Autodesk Inventor part; units mm, degrees
ref_plane "YZ Plane" through (0, 0, 0) normal (1, 0, 0) x (0, 1, 0)
ref_plane "XZ Plane" through (0, 0, 0) normal (0, 1, 0) x (-1, 0, 0)
ref_plane "XY Plane" through (0, 0, 0) normal (0, 0, 1) x (1, 0, 0)
sketch "Sketch1" plane through (0, 0, 0) normal (0, 1, 0) x (-1, 0, 0)
  line L0 (59.9595, 0.0507) -> (-0.0405, 0.0507)
  line L1 (-0.0405, 0.0507) -> (-0.0405, -59.9493)
  line L2 (-0.0405, -59.9493) -> (59.9595, -59.9493)
  line L3 (59.9595, -59.9493) -> (59.9595, 0.0507)
  line L4 (54, -52.088) -> (6, -52.088)
  line L5 (6, -52.088) -> (6, -50.088)
  line L6 (6, -50.088) -> (54, -50.088)
  line L7 (54, -50.088) -> (54, -52.088)
  line L8 (54, -46.088) -> (6, -46.088)
  line L9 (6, -46.088) -> (6, -44.088)
  line L10 (6, -44.088) -> (54, -44.088)
  line L11 (54, -44.088) -> (54, -46.088)
  line L12 (54, -40.088) -> (6, -40.088)
  line L13 (6, -40.088) -> (6, -38.088)
  line L14 (6, -38.088) -> (54, -38.088)
  line L15 (54, -38.088) -> (54, -40.088)
  line L16 (54, -34.088) -> (6, -34.088)
  line L17 (6, -34.088) -> (6, -32.088)
  line L18 (6, -32.088) -> (54, -32.088)
  line L19 (54, -32.088) -> (54, -34.088)
  line L20 (54, -28.0372) -> (6, -28.0372)
  line L21 (6, -28.0372) -> (6, -26.088)
  line L22 (6, -26.088) -> (54, -26.088)
  line L23 (54, -26.088) -> (54, -28.0372)
  line L24 (54, -22.088) -> (6, -22.088)
  line L25 (6, -22.088) -> (6, -20.088)
  line L26 (6, -20.088) -> (54, -20.088)
  line L27 (54, -20.088) -> (54, -22.088)
  line L28 (54, -16.088) -> (6, -16.088)
  line L29 (6, -16.088) -> (6, -14.088)
  line L30 (6, -14.088) -> (54, -14.088)
  line L31 (54, -14.088) -> (54, -16.088)
  line L32 (54, -10.088) -> (6, -10.088)
  line L33 (6, -10.088) -> (6, -8.088)
  line L34 (6, -8.088) -> (54, -8.088)
  line L35 (54, -8.088) -> (54, -10.088)
  line L36 (2, -58) -> (58, -58)
  line L37 (58, -58) -> (58, -2)
  line L38 (58, -2) -> (2, -2)
  line L39 (2, -2) -> (2, -58)
  point P0 (0, 0)
  dimension "d0" = 60
  dimension "d1" = 60
extrude "Bottom" add sketch "Sketch1" along normal blind 2 contours L3 L2 L1 L0 | L39 L38 L37 L36
sketch "Sketch2" plane through (0, 2, 0) normal (0, 1, 0) x (1, 0, 0)
  line L0 (-59.9595, -0.0507) -> (0.0405, -0.0507)
  line L1 (-60, 59.9493) -> (-58, 59.9493)
  line L2 (-58, 59.9493) -> (-58, -0.0507)
  line L3 (-58, -0.0507) -> (-60, -0.0507)
  line L4 (-60, -0.0507) -> (-60, 59.9493)
  line L5 (0.0405, 59.9493) -> (-59.9595, 59.9493)
  line L6 (-2, 59.9493) -> (0.0405, 59.9493)
  line L7 (0.0405, 59.9493) -> (0.0405, -0.0507)
  line L8 (0.0405, -0.0507) -> (-2, -0.0507)
  line L9 (-2, -0.0507) -> (-2, 59.9493)
  line L10 (-58, 59.9493) -> (-2, 59.9493)
  line L11 (-2, 59.9493) -> (-2, 58)
  line L12 (-2, 58) -> (-58, 58)
  line L13 (-58, 58) -> (-58, 59.9493)
  line L14 (-58, 2) -> (-2, 2)
  line L15 (-2, 2) -> (-2, -0.0507)
  line L16 (-2, -0.0507) -> (-58, -0.0507)
  line L17 (-58, -0.0507) -> (-58, 2)
  point P0 (-2, 2)
extrude "Walls" add sketch "Sketch2" along normal blind 26 contours L3 L4 L1 L2 L0 | L2 L14 L9 L0 | L9 L5 L7 L0 | L2 L5 L9 L12
sketch "Sketch3" plane through (-59.9595, 0, 0.0507) normal (0, 0, 1) x (1, 0, 0)
  line L0 (4, 4) -> (12, 4)
  line L1 (12, 4) -> (12, 14)
  line L2 (12, 14) -> (4, 14)
  line L3 (4, 14) -> (4, 4)
  line L4 (5.6179, 18.3587) -> (10.1248, 18.3587) construction
  line L5 (10.1248, 18.3587) -> (10.1248, 14.1529) construction
  line L6 (10.1248, 14.1529) -> (5.6179, 14.1529) construction
  line L7 (5.6179, 14.1529) -> (5.6179, 18.3587) construction
  circle A0 centre (38, 10) radius 3.6056
  line L8 (32.7887, 17.939) -> (43.0738, 17.939) construction
  line L9 (43.0738, 17.939) -> (43.0738, 14.8367) construction
  line L10 (43.0738, 14.8367) -> (32.7887, 14.8367) construction
  line L11 (32.7887, 14.8367) -> (32.7887, 17.939) construction
  point P0 (59.9595, 0)
extrude "AC/Reset" cut sketch "Sketch3" against normal blind 10
sketch "Sketch4" plane through (0, 28, 0) normal (0, 1, 0) x (1, 0, 0)
  line L0 (0.0405, -0.0507) -> (0.0405, 59.9493)
  line L1 (-59.9595, 60) -> (0.0405, 60)
  line L2 (0.0405, 60) -> (0.0405, -0.0507)
  line L3 (0.0405, -0.0507) -> (-59.9595, -0.0507)
  line L4 (-59.9595, -0.0507) -> (-59.9595, 60)
  circle A0 centre (-42, 42) radius 10
  line L5 (-6, 32.088) -> (-54, 32.088)
  line L6 (-23, 52) -> (-8, 52)
  line L7 (-8, 52) -> (-8, 32.088)
  line L8 (-8, 32.088) -> (-23, 32.088)
  line L9 (-23, 32.088) -> (-23, 52)
  point P0 (0, 0)
  dimension "d8" = 20
  dimension "d9" = 60
extrude "Extrusion4" add sketch "Sketch4" along normal blind 2
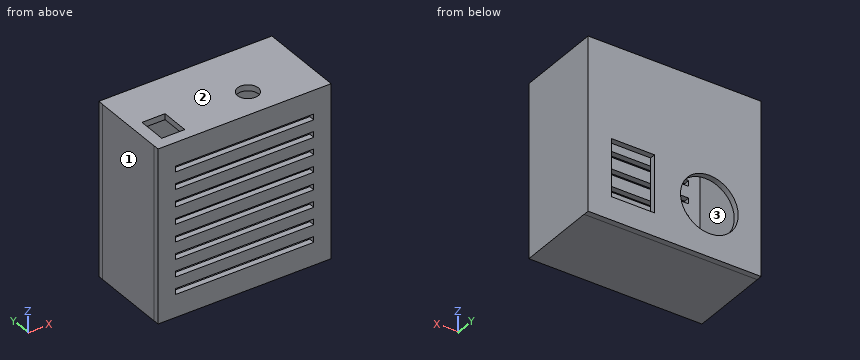
Geometry check sheet. Reference: the model listing, model coordinates, mm. Face numbers are marked on the shaded views. Give positions to 0.01 mm unless a question says otherwise; leave off trailing zeros. Order: outer loops, then holes, each group sorted by start corner. A loop starts at its lowest first (then second) coordinate and runs counter-clockwise, first axis right, second up. Notation, with made-up numbers: (6, -31) - (51, -31) arc R9 cw to (51, -16) - close; hole circle Ø10 at (30.5, 69). An arc over 180 degrees is marked (long way). Write item = value, one per line. Start each with the question number.
1) Section check B-B (x = -5). Enter the section's corners in (y, z).
2) Section check C-C (y = 10). Enter the section's corners in (x, z).
3) Gauge pin test, flat ends, axial feed: pin 1 Ø8 at (x, y) = (-50.5, 13) entering from -Z; pin 2 Ø0.6 at (y, z) = (28.5, -35) entering from -X. Record the tip position at first contact, or that the pin passes through.
4) Draft check along Z on the marked faces 1, 2 and 3. Enter one of: released by +Z, released by -Z, zero draft, split by the parting line, or undercut.
5) Section check D-D (z = -54). Enter the section's corners in (x, y).
6) Scan lines: L1, parallel to X at y = 7.25, z = -54.5; L2, parallel to Z at x = -14, y = 20.75; L3, parallel to Y at x = -24, z = -55.5. Record each from-to range of solid material in increasing order.
7) Section check A-A (z = -42). Enter the section's corners in (x, y), then the cut area to 3 significant figures.
Geometry check:
q1.outline = (0, -59.95) - (28, -59.95) - (28, -60) - (30, -60) - (30, 0.05) - (0, 0.05) - close; hole (2, -58) - (28, -58) - (28, -2) - (2, -2) - close
q2.outline = (-60, -59.95) - (0.04, -59.95) - (0.04, 0.05) - (-18.35, 0.05) - (-18.35, -2) - (-2, -2) - (-2, -58) - (-58, -58) - (-58, -2) - (-55.96, -2) - (-55.96, 0.05) - (-60, 0.05) - close; (-47.96, -2) - (-25.57, -2) - (-25.57, 0.05) - (-47.96, 0.05) - close
q3.pin_1 = -59.95
q3.pin_2 = -59.96
q4.face_1 = zero draft
q4.face_2 = released by +Z
q4.face_3 = undercut
q5.outline = (-60, 2) - (-59.96, 2) - (-59.96, 0) - (0.04, 0) - (0.04, 30) - (-59.96, 30) - (-59.96, 28) - (-60, 28) - close; hole (-58, 2) - (-2, 2) - (-2, 28) - (-58, 28) - close
q6.L1 = -60 to -58, -2 to 0.04
q6.L2 = -59.95 to -58, -2 to 0.05
q6.L3 = 0 to 2, 28 to 30
q7.outline = (-60, 2) - (-59.96, 2) - (-59.96, 0) - (0.04, 0) - (0.04, 30) - (-8, 30) - (-8, 28) - (-2, 28) - (-2, 2) - (-58, 2) - (-58, 28) - (-52, 28) - (-52, 30) - (-59.96, 30) - (-59.96, 28) - (-60, 28) - close; (-32, 28) - (-23, 28) - (-23, 30) - (-32, 30) - close
q7.area = 275 mm2
